from build123d import *

# Parameters (mm, degrees)
CYLINDER067_R             = 1.75
CYLINDER067_DEPTH         = 22
CYLINDER067_PITCH_ANGLE   = 90
CYLINDER061_R             = 1.25
CYLINDER061_DEPTH         = 22
CYLINDER061_PITCH_ANGLE   = 90
CYLINDER062_R             = 1.25
CYLINDER062_DEPTH         = 22
CYLINDER062_PITCH_ANGLE   = 90
CYLINDER060_R             = 1.25
CYLINDER060_DEPTH         = 22
CYLINDER060_PITCH_ANGLE   = 90
CYLINDER059_R             = 1.25
CYLINDER059_DEPTH         = 22
CYLINDER059_PITCH_ANGLE   = 90
CYLINDER065_R             = 1.25
CYLINDER065_DEPTH         = 22
CYLINDER065_PITCH_ANGLE   = 90
CYLINDER066_R             = 1.25
CYLINDER066_DEPTH         = 22
CYLINDER066_PITCH_ANGLE   = 90
CYLINDER064_R             = 1.25
CYLINDER064_DEPTH         = 22
CYLINDER064_PITCH_ANGLE   = 90
CYLINDER063_R             = 1.25
CYLINDER063_DEPTH         = 22
CYLINDER063_PITCH_ANGLE   = 90
FUSION047_ROLL_ANGLE      = 34
FUSION047_PLACEMENT_ANGLE = -90
CYLINDER058_R             = 3
CYLINDER058_DEPTH         = 22
CYLINDER058_PITCH_ANGLE   = 90
CYLINDER057_R             = 3
CYLINDER057_DEPTH         = 13
CYLINDER057_ROLL_ANGLE    = 90
CYLINDER056_R             = 10
CYLINDER056_DEPTH         = 10
CYLINDER056_ROLL_ANGLE    = 90
PAD007_DEPTH              = 34
PAD005_DEPTH              = 42
CHAMFER104_SIZE           = 5
CHAMFER105_SIZE           = 5


with BuildPart() as cilindro011:
    # Cylinder067 → Cylinder067 (new body)
    with BuildSketch(Plane.XY):
        Circle(CYLINDER067_R)
    extrude(amount=CYLINDER067_DEPTH)


with BuildPart() as cilindro011_1:
    # Cylinder067 pitch: moved
    add(cilindro011.part.rotate(Axis((0, 0, 0), (0, 1, 0)), CYLINDER067_PITCH_ANGLE))


with BuildPart() as cilindro011_2:
    # Cylinder067 placement: moved
    add(cilindro011_1.part.moved(Location((-4.75, -32, 125.75))))


with BuildPart() as cilindro005:
    # Cylinder061 → Cylinder061 (new body)
    with BuildSketch(Plane.XY):
        Circle(CYLINDER061_R)
    extrude(amount=CYLINDER061_DEPTH)


with BuildPart() as cilindro005_1:
    # Cylinder061 pitch: moved
    add(cilindro005.part.rotate(Axis((0, 0, 0), (0, 1, 0)), CYLINDER061_PITCH_ANGLE))


with BuildPart() as cilindro005_2:
    # Cylinder061 placement: moved
    add(cilindro005_1.part.moved(Location((20.25, -38, 124.25))))


with BuildPart() as cilindro006:
    # Cylinder062 → Cylinder062 (new body)
    with BuildSketch(Plane.XY):
        Circle(CYLINDER062_R)
    extrude(amount=CYLINDER062_DEPTH)


with BuildPart() as cilindro006_1:
    # Cylinder062 pitch: moved
    add(cilindro006.part.rotate(Axis((0, 0, 0), (0, 1, 0)), CYLINDER062_PITCH_ANGLE))


with BuildPart() as cilindro006_2:
    # Cylinder062 placement: moved
    add(cilindro006_1.part.moved(Location((20.25, -26, 127.25))))


with BuildPart() as cilindro004:
    # Cylinder060 → Cylinder060 (new body)
    with BuildSketch(Plane.XY):
        Circle(CYLINDER060_R)
    extrude(amount=CYLINDER060_DEPTH)


with BuildPart() as cilindro004_1:
    # Cylinder060 pitch: moved
    add(cilindro004.part.rotate(Axis((0, 0, 0), (0, 1, 0)), CYLINDER060_PITCH_ANGLE))


with BuildPart() as cilindro004_2:
    # Cylinder060 placement: moved
    add(cilindro004_1.part.moved(Location((20.25, -30, 118.75))))


with BuildPart() as fusion046:
    # Cylinder059 → Cylinder059 (new body)
    with BuildSketch(Plane.XY):
        Circle(CYLINDER059_R)
    extrude(amount=CYLINDER059_DEPTH)


with BuildPart() as fusion046_1:
    # Cylinder059 pitch: moved
    add(fusion046.part.rotate(Axis((0, 0, 0), (0, 1, 0)), CYLINDER059_PITCH_ANGLE))


with BuildPart() as fusion046_2:
    # Cylinder059 placement: moved
    add(fusion046_1.part.moved(Location((20.25, -34, 132.75))))

    # Fusion046: union Cilindro005, Cilindro006, Cilindro004
    add(cilindro005_2.part)
    add(cilindro006_2.part)
    add(cilindro004_2.part)


with BuildPart() as cilindro009:
    # Cylinder065 → Cylinder065 (new body)
    with BuildSketch(Plane.XY):
        Circle(CYLINDER065_R)
    extrude(amount=CYLINDER065_DEPTH)


with BuildPart() as cilindro009_1:
    # Cylinder065 pitch: moved
    add(cilindro009.part.rotate(Axis((0, 0, 0), (0, 1, 0)), CYLINDER065_PITCH_ANGLE))


with BuildPart() as cilindro009_2:
    # Cylinder065 placement: moved
    add(cilindro009_1.part.moved(Location((20.25, -38, 124.25))))


with BuildPart() as cilindro010:
    # Cylinder066 → Cylinder066 (new body)
    with BuildSketch(Plane.XY):
        Circle(CYLINDER066_R)
    extrude(amount=CYLINDER066_DEPTH)


with BuildPart() as cilindro010_1:
    # Cylinder066 pitch: moved
    add(cilindro010.part.rotate(Axis((0, 0, 0), (0, 1, 0)), CYLINDER066_PITCH_ANGLE))


with BuildPart() as cilindro010_2:
    # Cylinder066 placement: moved
    add(cilindro010_1.part.moved(Location((20.25, -26, 127.25))))


with BuildPart() as cilindro008:
    # Cylinder064 → Cylinder064 (new body)
    with BuildSketch(Plane.XY):
        Circle(CYLINDER064_R)
    extrude(amount=CYLINDER064_DEPTH)


with BuildPart() as cilindro008_1:
    # Cylinder064 pitch: moved
    add(cilindro008.part.rotate(Axis((0, 0, 0), (0, 1, 0)), CYLINDER064_PITCH_ANGLE))


with BuildPart() as cilindro008_2:
    # Cylinder064 placement: moved
    add(cilindro008_1.part.moved(Location((20.25, -30, 118.75))))


with BuildPart() as fusion047:
    # Cylinder063 → Cylinder063 (new body)
    with BuildSketch(Plane.XY):
        Circle(CYLINDER063_R)
    extrude(amount=CYLINDER063_DEPTH)


with BuildPart() as fusion047_1:
    # Cylinder063 pitch: moved
    add(fusion047.part.rotate(Axis((0, 0, 0), (0, 1, 0)), CYLINDER063_PITCH_ANGLE))


with BuildPart() as fusion047_2:
    # Cylinder063 placement: moved
    add(fusion047_1.part.moved(Location((20.25, -34, 132.75))))

    # Fusion047: union Cilindro009, Cilindro010, Cilindro008
    add(cilindro009_2.part)
    add(cilindro010_2.part)
    add(cilindro008_2.part)


with BuildPart() as fusion047_3:
    # Fusion047 roll: moved
    add(fusion047_2.part.rotate(Axis((0, 0, 0), (1, 0, 0)), FUSION047_ROLL_ANGLE))


with BuildPart() as fusion047_4:
    # Fusion047 placement: moved
    add(fusion047_3.part.moved(Location((114.107998, 21, 33.646227))).rotate(Axis((114.107998, 21, 33.646227), (0, 0, 1)), FUSION047_PLACEMENT_ANGLE))


with BuildPart() as cilindro002:
    # Cylinder058 → Cylinder058 (new body)
    with BuildSketch(Plane.XY):
        Circle(CYLINDER058_R)
    extrude(amount=CYLINDER058_DEPTH)


with BuildPart() as cilindro002_1:
    # Cylinder058 pitch: moved
    add(cilindro002.part.rotate(Axis((0, 0, 0), (0, 1, 0)), CYLINDER058_PITCH_ANGLE))


with BuildPart() as cilindro002_2:
    # Cylinder058 placement: moved
    add(cilindro002_1.part.moved(Location((20.25, -32, 125.75))))


with BuildPart() as cilindro001:
    # Cylinder057 → Cylinder057 (new body)
    with BuildSketch(Plane.XY):
        Circle(CYLINDER057_R)
    extrude(amount=CYLINDER057_DEPTH)


with BuildPart() as cilindro001_1:
    # Cylinder057 roll: moved
    add(cilindro001.part.rotate(Axis((0, 0, 0), (1, 0, 0)), CYLINDER057_ROLL_ANGLE))


with BuildPart() as cilindro001_2:
    # Cylinder057 placement: moved
    add(cilindro001_1.part.moved(Location((17.25, -6, 120))))


with BuildPart() as cilindro:
    # Cylinder056 → Cylinder056 (new body)
    with BuildSketch(Plane.XY):
        Circle(CYLINDER056_R)
    extrude(amount=CYLINDER056_DEPTH)


with BuildPart() as cilindro_1:
    # Cylinder056 roll: moved
    add(cilindro.part.rotate(Axis((0, 0, 0), (1, 0, 0)), CYLINDER056_ROLL_ANGLE))


with BuildPart() as cilindro_2:
    # Cylinder056 placement: moved
    add(cilindro_1.part.moved(Location((17.25, -4, 120))))


with BuildPart() as pad007:
    # Sketch012 → Pad007 (new body)
    with BuildSketch(Plane(origin=(3, -12, -1), x_dir=(0, 1, 0), z_dir=(1, 0, 0))):
        Polygon((-4.882067, 101.940956), (-4.882067, 138.559921), (-40.571098, 142.373672), (-40.571098, 120.688431), align=None)
    extrude(amount=PAD007_DEPTH)


with BuildPart() as obj1:
    # Sketch010 → Pad005 (new body)
    with BuildSketch(Plane.YZ.offset(-1)):
        Polygon((-7.053021, 102.221077), (-7.053021, 138.840042), (-42.260719, 142.653793), (-42.260719, 119.265137), align=None)
    extrude(amount=PAD005_DEPTH)

    # Cut085: cut Pad007
    add(pad007.part, mode=Mode.SUBTRACT)

    # Cut086: cut Cilindro
    add(cilindro_2.part, mode=Mode.SUBTRACT)

    # Cut087: cut Cilindro001
    add(cilindro001_2.part, mode=Mode.SUBTRACT)

    # Chamfer104
    chamfer104_edges = [obj1.edges().sort_by_distance(p)[0] for p in [
        (20, -16.882067, 106.979322),
    ]]
    chamfer(chamfer104_edges, length=CHAMFER104_SIZE)

    # Cut088: cut Cilindro002
    add(cilindro002_2.part, mode=Mode.SUBTRACT)

    # Cut089: cut Fusion047
    add(fusion047_4.part, mode=Mode.SUBTRACT)

    # Cut090: cut Fusion046
    add(fusion046_2.part, mode=Mode.SUBTRACT)

    # Cut091: cut Cilindro011
    add(cilindro011_2.part, mode=Mode.SUBTRACT)

    # Chamfer105
    chamfer105_edges = [obj1.edges().sort_by_distance(p)[0] for p in [
        (41, -7.053021, 120.530559),
    ]]
    chamfer(chamfer105_edges, length=CHAMFER105_SIZE)


solid = obj1.part
Read the model definition and answer for the solid it produces. Units are mm, in the model's axes. A direction names the side the tool comes from. Round coordinates to 2 decimals unless told otherwise and drop trailing zeros. Write each loop counter-clockwise with the first axis right and the second up, starting at its lowest first coordinate (ties: lowest second). Pieces come first, ordered by that corner, then holes.
Q1. The mould has two halves that part along Y. Classify faces 5 (the face through (13.31, -15.42, 116.64)), 6 (the face through (19.762, -14.663, 108.44)), 7 (the face through (39, -38, 123)): released by +Y, released by -Y, zero draft, split by the parting line, or undercut.
Values:
face 5: zero draft
face 6: released by -Y
face 7: undercut
Q2. Find section A-A on x = 17.25. Determine the outline of the cut face in (y, z).
Values:
outline: (-42.26, 140.27) - (-16.88, 137.56) - (-16.88, 123) - (-14, 123) - (-14, 130) - (-7.05, 130) - (-7.05, 138.84) - (-42.26, 142.65) - close; (-16.88, 111.98) - (-12.38, 104.8) - (-7.05, 102.22) - (-7.05, 110) - (-14, 110) - (-14, 117) - (-16.88, 117) - close
Q3. Straight lines are drawn through the part: line 1 (X direction, y = -24, z = 120); line 2 (Z direction, x = 17, y = -10); line 3 (Y direction, x = 39.55, z = 132.75). For each, find the intervals that lie inside material, in ascending order.
Values:
line 1: x = -1 to 3, 37 to 41
line 2: z = 103.65 to 110, 130 to 139.16
line 3: y = -42.26 to -35.25, -32.75 to -10.6
Q4. Flat-ended cylindrical pins translate along their axes: P1, Ø5, axis at x = 9.5, z = 118.5, coming from the -Y side; P2, Ø3, axis at y = -32, z = 125.75, coming from the +X side; P3, Ø8, axis at x = 31, z = 138, coming from the -Y side; P4, Ø16, axis at x = 17.25, z = 120, coming from the +Y side. Find the tip coordinate at first contact, or state that the pin passes through.
Values:
P1: stops at y = -16.88
P2: passes through
P3: stops at y = -42.26
P4: stops at y = -14
Q5. Find section D-D on x = 4.5. Determine the outline of the cut face in (y, z).
Values:
outline: (-42.26, 140.27) - (-16.88, 137.56) - (-16.88, 111.98) - (-12.38, 104.8) - (-7.05, 102.22) - (-7.05, 138.84) - (-42.26, 142.65) - close
Q6. Find section B-B on y = -38. Determine the outline of the cut face in (x, z), and give its area (3 significant figures).
Values:
outline: (-1, 117.2) - (3, 117.2) - (3, 139.82) - (37, 139.82) - (37, 125.5) - (41, 125.5) - (41, 142.19) - (-1, 142.19) - close; (37, 117.2) - (41, 117.2) - (41, 123) - (37, 123) - close
area: 271 mm2
Q7. A tool of negligible diameter and unlimited length cuts with its end or side. For faces 1 (the face through (22.63, -10.48, 128.43)), 2 (the face through (37, -28, 127)), 3 (the face through (39, -26, 126)), 4 (the face through (41, -27.4, 128.1)), from which of +Z, -Z, +X, -X, +Y, -Y can it reach the whole face along a straight path? Write none if from no direction.
Values:
face 1: +Y
face 2: -Z, -Y
face 3: +X
face 4: +Z, -Z, +X, +Y, -Y
Q8. Find section C-C on z = 132.75. Determine the outline of the cut face in (x, y).
Values:
outline: (-1, -42.26) - (3, -42.26) - (3, -16.88) - (37, -16.88) - (37, -32.75) - (41, -32.75) - (41, -12.05) - (36, -7.05) - (-1, -7.05) - close; (37, -42.26) - (41, -42.26) - (41, -35.25) - (37, -35.25) - close
